The model under review builds one solid part; all positions refer to its coordinate system, in mm. Round coordinates to 2 decimals unless told otherwise and drop trailing zeros. Order: outer loops, then holes, each group sorted by start corner. A loop starts at its lowest first (then second) coordinate and runs counter-clockwise, first axis right, second up.
1) Consider section B-B (y = 61). Give the boundary of the cut face in (x, z).
2) Clearance check with a flat-ended pin moving along its axis: P1, Ø11, axis at x = 200, y = 0, coming from the +Z side. State where the tip first meets the part, or that it passes through.
3) To check wall thickness, follow L1, parallel to X at y = 31, z = 0.75; L2, parallel to Y at x = 31, z = 0.35; L3, parallel to Y at x = 97.5, z = 0.5. State the ranges of each line that lie inside material, in increasing order.
4) Consider section C-C (z = 0.25). Give the number of separate pieces and of enclosed holes in the cut face, then the cut area to 3 significant figures.
5) Mouldability with a two-part tool opening along X and no side actions: class faces 1 (the face through (-3, -17, 0)), 2 (the face through (-196.66, 1.05, 0.49)) as pulls with the +X half, pulls with the -X half, needs draft (parallel to the pull), parting line crosses it, or undercut.
6) Consider section D-D (x = -92). Give the boundary of the cut face in (y, z).
7) Consider section A-A (x = -1). Give the boundary of the cut face in (y, z).
from build123d import *

# Parameters (mm, degrees)
ESQUISSE1_R        = 26.5
ESQUISSE1_R_2      = 2.5
ESQUISSE1_R_3      = 5
ESQUISSE1_R_4      = 11
ESQUISSE1_R_5      = 6
ESQUISSE1_R_6      = 3.5
ESQUISSE1_W        = 89
ESQUISSE1_H        = 28
BOSS_EXTRU_1_DEPTH = 1


with BuildPart() as part:
    # Esquisse1 → Boss.-Extru.1 (new body)
    with BuildSketch(Plane.XY):
        with BuildLine():
            Line((205, 80), (-205, 80))
            ThreePointArc((-205, 80), (-208.535533906, 78.535533906), (-210, 75))
            Line((-210, 75), (-210, -75))
            ThreePointArc((-210, -75), (-208.535533906, -78.535533906), (-205, -80))
            Line((-205, -80), (205, -80))
            ThreePointArc((205, -80), (208.535533906, -78.535533906), (210, -75))
            Line((210, -75), (210, 75))
            ThreePointArc((210, 75), (208.535533906, 78.535533906), (205, 80))
        make_face()
        with Locations((-161, 30)):
            Circle(ESQUISSE1_R, mode=Mode.SUBTRACT)
        with Locations((-97, 30)):
            Circle(ESQUISSE1_R, mode=Mode.SUBTRACT)
        with Locations((-33, 30)):
            Circle(ESQUISSE1_R, mode=Mode.SUBTRACT)
        with Locations((31, 30)):
            Circle(ESQUISSE1_R, mode=Mode.SUBTRACT)
        with Locations((74, 40)):
            Circle(ESQUISSE1_R_2, mode=Mode.SUBTRACT)
        with Locations((74, 0)):
            Circle(ESQUISSE1_R_2, mode=Mode.SUBTRACT)
        with Locations((177, 0)):
            Circle(ESQUISSE1_R_2, mode=Mode.SUBTRACT)
        with Locations((177, 40)):
            Circle(ESQUISSE1_R_2, mode=Mode.SUBTRACT)
        with Locations((31, -32)):
            Circle(ESQUISSE1_R, mode=Mode.SUBTRACT)
        with Locations((-129, 61)):
            Circle(ESQUISSE1_R_3, mode=Mode.SUBTRACT)
        with Locations((-65, 61)):
            Circle(ESQUISSE1_R_3, mode=Mode.SUBTRACT)
        with Locations((-1, 61)):
            Circle(ESQUISSE1_R_3, mode=Mode.SUBTRACT)
        with Locations((-1, -1)):
            Circle(ESQUISSE1_R_3, mode=Mode.SUBTRACT)
        with Locations((-65, -1)):
            Circle(ESQUISSE1_R_3, mode=Mode.SUBTRACT)
        with Locations((-129, -1)):
            Circle(ESQUISSE1_R_3, mode=Mode.SUBTRACT)
        with Locations((-181, -40)):
            Circle(ESQUISSE1_R_4, mode=Mode.SUBTRACT)
        with Locations((-152, -40)):
            Circle(ESQUISSE1_R_5, mode=Mode.SUBTRACT)
        with Locations((200, 0)):
            Circle(ESQUISSE1_R_6, mode=Mode.SUBTRACT)
        with Locations((-200, 0)):
            Circle(ESQUISSE1_R_6, mode=Mode.SUBTRACT)
        with Locations((-132, -40)):
            Circle(ESQUISSE1_R_5, mode=Mode.SUBTRACT)
        with Locations((-112, -40)):
            Circle(ESQUISSE1_R_5, mode=Mode.SUBTRACT)
        with Locations((-92, -40)):
            Circle(ESQUISSE1_R_5, mode=Mode.SUBTRACT)
        with Locations((-72, -40)):
            Circle(ESQUISSE1_R_5, mode=Mode.SUBTRACT)
        with Locations((-52, -40)):
            Circle(ESQUISSE1_R_5, mode=Mode.SUBTRACT)
        with Locations((-32, -40)):
            Circle(ESQUISSE1_R_5, mode=Mode.SUBTRACT)
        with Locations((-12, -40)):
            Circle(ESQUISSE1_R_5, mode=Mode.SUBTRACT)
        with Locations((125.5, 40)):
            Rectangle(ESQUISSE1_W, ESQUISSE1_H, mode=Mode.SUBTRACT)
        with Locations((125.5, 0)):
            Rectangle(ESQUISSE1_W, ESQUISSE1_H, mode=Mode.SUBTRACT)
    extrude(amount=BOSS_EXTRU_1_DEPTH)


solid = part.part
Answer below:
1. outline: (-210, 0) - (-134, 0) - (-134, 1) - (-210, 1) - close; (-124, 0) - (-70, 0) - (-70, 1) - (-124, 1) - close; (-60, 0) - (-6, 0) - (-6, 1) - (-60, 1) - close; (4, 0) - (210, 0) - (210, 1) - (4, 1) - close
2. P1: stops at z = 1
3. L1: x = -210 to -187.48, -134.52 to -123.48, -70.52 to -59.48, -6.52 to 4.52, 57.48 to 81, 170 to 210
3. L2: y = -80 to -58.5, -5.5 to 3.5, 56.5 to 80
3. L3: y = -80 to -14, 14 to 26, 54 to 80
4. separate pieces: 1
4. enclosed holes: 28
4. area: 49,300 mm2
5. face 1: needs draft
5. face 2: undercut
6. outline: (-80, 0) - (-46, 0) - (-46, 1) - (-80, 1) - close; (-34, 0) - (3.98, 0) - (3.98, 1) - (-34, 1) - close; (56.02, 0) - (80, 0) - (80, 1) - (56.02, 1) - close
7. outline: (-80, 0) - (-6, 0) - (-6, 1) - (-80, 1) - close; (4, 0) - (56, 0) - (56, 1) - (4, 1) - close; (66, 0) - (80, 0) - (80, 1) - (66, 1) - close
